Autodesk Inventor part; units mm, degrees
ref_plane "YZ Plane" through (0, 0, 0) normal (1, 0, 0) x (0, 1, 0)
ref_plane "XZ Plane" through (0, 0, 0) normal (0, 1, 0) x (-1, 0, 0)
ref_plane "XY Plane" through (0, 0, 0) normal (0, 0, 1) x (1, 0, 0)
sketch "Sketch1" plane through (0, 0, 0) normal (1, 0, 0) x (0, 1, 0)
  line L0 (0, 0) -> (0, -30)
  line L1 (13.5, 0) -> (30, 0) construction
  line L2 (0, -30) -> (85, -30)
  line L3 (13.5, 0) -> (85, 0)
  line L4 (85, 0) -> (85, -30)
  line L5 (0, 0) -> (0, 10.5)
  line L6 (13.5, 0) -> (14, 0) construction
  line L7 (0, 10.5) -> (8.5, 10.5)
  line L8 (8.5, 10.5) -> (8.5, 30.5)
  line L9 (8.5, 30.5) -> (13.5, 30.5)
  line L10 (13.5, 30.5) -> (13.5, 0)
  point P0 (0, -15)
  dimension "d0" = 30
  dimension "d2" = 85
  dimension "d4" = 10.5
  dimension "d6" = 8.5
  dimension "d7" = 20
  dimension "d8" = 5
  dimension "d47" = 30
extrude "Extrusion1" add sketch "Sketch1" along normal blind 30
sketch "Sketch2" plane through (0, 85, 0) normal (0, 1, 0) x (1, 0, 0)
  line L0 (4.5, 4.5) -> (4.5, 25.5)
  line L1 (4.5, 4.5) -> (25.5, 4.5) construction
  line L2 (4.5, 25.5) -> (25.5, 25.5)
  line L3 (25.5, 25.5) -> (25.5, 4.5)
  line L4 (25.5, 4.5) -> (4.5, 4.5)
  line L5 (30, 30) -> (30, 0)
  point P0 (0, 0)
  dimension "d13" = 21
  dimension "d14" = 90
  dimension "d15" = 21
  dimension "d16" = 90
  dimension "d17" = 21
  dimension "d18" = 90
  dimension "d19" = 21
  dimension "d46" = 4.5
  dimension "d48" = 90
  dimension "d49" = 4.5
extrude "Extrusion2" cut sketch "Sketch2" against normal blind 80
fillet "Fillet1" radius 2 12 edges at (30, 85, -15) (15, 85, 0) (15, 85, -30) (0, 85, -15) (30, 49.25, 0) (30, 42.5, -30) (0, 49.25, 0) (0, 42.5, -30) (0, 13.5, 15.25) (15, 13.5, 30.5) (30, 13.5, 15.25) (15, 13.5, 0)
sketch "Sketch4" plane through (2, 13.5, 2) normal (0, 1, 0) x (1, 0, 0)
  line L0 (-2, -28.5) -> (28, -28.5)
  point P0 (-2, 2)
  point P1 (13, -18.5)
  point P2 (13, -28.5)
  dimension "d37" = 10
hole "Hole1" at (15, 13.5, 20.5) direction (0, -1, 0) diameter 5 end through all countersink diameter 10 countersink angle 77.33
sketch "Sketch6" plane through (30, 0, 0) normal (1, 0, 0) x (0, 0, -1)
  line L0 (-10.5, 0) -> (28, 0)
  point P0 (0, 0)
  point P1 (15, 59)
  point P2 (15, 0)
  dimension "d45" = 59
hole "Hole2" at (30, 59, -15) direction (-1, 0, 0) diameter 5 end through all
chamfer "Chamfer2" distance 2 angle 45 4 edges at (4.5, 85, -15) (15, 85, -25.5) (25.5, 85, -15) (15, 85, -4.5)
fillet "Fillet3" radius 2 4 edges at (3.5, 84, -26.5) (26.5, 84, -26.5) (26.5, 84, -3.5) (3.5, 84, -3.5)
properties part number "flexibler_standfuß_v0.9"
For this review, take the finished solid that the model builds, in its own axes (mm). A direction names the side the tool comes from. Coordinates: 2 decimals unless noted, no trailing zeros. Write each loop counter-clockwise with the first axis right and the second up, starting at its lowest first coordinate (ties: lowest second). Pieces come first, ordered by that corner, then holes. Notation, with made-up numbers: (55, 41.25) -> (102, 41.25) arc R31 cw to (102, 77.25) -> close; hole circle Ø9 at (19.25, 55.25). An arc over 180 degrees is marked (long way). Put each result on its own line as item: value.
Q1. Take a section at D-D, the plane y = 23. State the section outline as (x, z) points.
From the geometry:
outline: (0, -28) arc R2 ccw to (2, -30) -> (28, -30) arc R2 ccw to (30, -28) -> (30, -2) arc R2 ccw to (28, 0) -> (2, 0) arc R2 ccw to (0, -2) -> close; hole (4.5, -25.5) -> (25.5, -25.5) -> (25.5, -4.5) -> (4.5, -4.5) -> close
Q2. Clearance check with flat-ended pins moving along their axes: pin 1 Ø2.5 at (x, y) = (11.5, 3.5) entering from +Z; pin 2 Ø1 at (x, y) = (16, 17) entering from +Z; pin 3 Ø16 at (x, z) = (17.5, 20) entering from -Y. State where each tip first meets the part, or that it passes through.
From the geometry:
pin 1: stops at z = 10.5
pin 2: stops at z = 0
pin 3: stops at y = 8.5
Q3. Take a section at C-C, the plane z = 20.5. State the section outline as (x, y) points, then the cut area to 3 significant figures.
From the geometry:
outline: (0, 8.5) -> (12.5, 8.5) -> (12.5, 10.38) -> (10, 13.5) -> (2, 13.5) arc R2 ccw to (0, 11.5) -> close; (17.5, 8.5) -> (30, 8.5) -> (30, 11.5) arc R2 ccw to (28, 13.5) -> (20, 13.5) -> (17.5, 10.38) -> close
area: 115 mm2
Q4. Take a section at B-B, the plane x = 15. State the section outline as (y, z) points, then the cut area to 3 significant figures.
From the geometry:
outline: (0, -30) -> (83, -30) arc R2 ccw to (85, -28) -> (85, -27.5) -> (83, -25.5) -> (5, -25.5) -> (5, -4.5) -> (83, -4.5) -> (85, -2.5) -> (85, -2) arc R2 ccw to (83, 0) -> (15.5, 0) arc R2 cw to (13.5, 2) -> (13.5, 15.5) -> (10.38, 18) -> (8.5, 18) -> (8.5, 10.5) -> (0, 10.5) -> close; (8.5, 23) -> (10.38, 23) -> (13.5, 25.5) -> (13.5, 28.5) arc R2 ccw to (11.5, 30.5) -> (8.5, 30.5) -> close
area: 1,070 mm2
Q5. Wall thickness on L1, parallel to Z at x = 15, y = 9.3; L2, parallel to Z at x = 17.25, y = 34; L3, parallel to X at y = 40.5, z = -19: over which ranges is each line inside the solid? List them lowest first.
From the geometry:
L1: z = -30 to -25.5, -4.5 to 18, 23 to 30.5
L2: z = -30 to -25.5, -4.5 to 0
L3: x = 0 to 4.5, 25.5 to 30
Q6. The part is to be moulded in two halves that separate along X. For faces 1 (the flat face through (15.2, 84, -26.5)), 2 (the cylindrical face through (0.57, 49.72, -0.6)), 3 (the cylindrical face through (15.21, 12.93, 29.9)), 4 (the cylindrical face through (25.99, 83.88, -26.01)), say which applies: +X half, -X half, draft (parallel to the pull), parting line (faces both ways), or undercut.
From the geometry:
face 1: undercut
face 2: -X half
face 3: draft
face 4: undercut
Q7. Take a section at A-A, the plane y = 59. State the section outline as (x, z) points.
From the geometry:
outline: (0, -28) arc R2 ccw to (2, -30) -> (28, -30) arc R2 ccw to (30, -28) -> (30, -17.5) -> (25.5, -17.5) -> (25.5, -25.5) -> (4.5, -25.5) -> (4.5, -17.5) -> (0, -17.5) -> close; (0, -12.5) -> (4.5, -12.5) -> (4.5, -4.5) -> (25.5, -4.5) -> (25.5, -12.5) -> (30, -12.5) -> (30, -2) arc R2 ccw to (28, 0) -> (2, 0) arc R2 ccw to (0, -2) -> close
Q8. Tool access review of faces 5 (the flat face through (11, 8.5, 20)), 6 (the flat face through (14.8, 84, -3.5)), 7 (the flat face through (0, 41, -11)): name each direction out of +Z, -Z, +X, -X, +Y, -Y from which nothing blocks a thin tool from reaching the whole face with its end or side.
From the geometry:
face 5: +Z, +X, -X, -Y
face 6: +Y
face 7: +Z, -Z, -X, +Y, -Y
